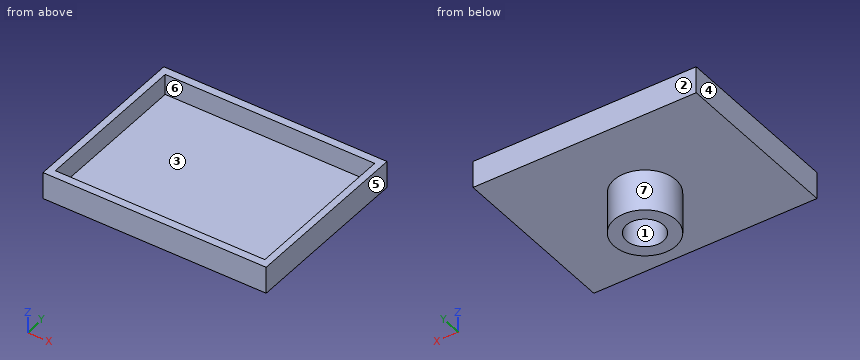
from build123d import *

# Parameters (mm, degrees)
ESQUISSE1_R             = 7.5
ESQUISSE1_R_2           = 4.5
BOSS_EXTRU_1_DEPTH      = 10
ESQUISSE2_W             = 54
ESQUISSE2_H             = 42
BOSS_EXTRU_2_DEPTH      = 6.5
ESQUISSE4_W             = 50.7
ESQUISSE4_H             = 38.2
ENL_V_MAT_EXTRU_2_DEPTH = 5


with BuildPart() as part:
    # Esquisse1 → Boss.-Extru.1 (new body)
    with BuildSketch(Plane.XY):
        Circle(ESQUISSE1_R)
        Circle(ESQUISSE1_R_2, mode=Mode.SUBTRACT)
    extrude(amount=BOSS_EXTRU_1_DEPTH)

    # Esquisse2 → Boss.-Extru.2 (add)
    with BuildSketch(Plane.XY.offset(10)):
        Rectangle(ESQUISSE2_W, ESQUISSE2_H)
    extrude(amount=BOSS_EXTRU_2_DEPTH)

    # Esquisse4 → Enlèv. mat.-Extru.2 (cut)
    with BuildSketch(Plane.XY.offset(16.5)):
        Rectangle(ESQUISSE4_W, ESQUISSE4_H)
    extrude(amount=-ENL_V_MAT_EXTRU_2_DEPTH, mode=Mode.SUBTRACT)


solid = part.part
Can you work these out from the model? Positions are in its coordinate system, mm. Face numbers are marked on the shaded views. A direction names the side the tool comes from. Round coordinates to 2 decimals unless told otherwise and drop trailing zeros. Order: outer loops, then holes, each group sorted by start corner. A loop starts at its lowest first (then second) coordinate and runs counter-clockwise, first axis right, second up. Notation, with made-up numbers: (-28.5, 23.5) -> (5.5, 23.5) arc R5 cw to (5.5, 30.5) -> close; hole circle Ø11 at (32, -31.75). An arc over 180 degrees is marked (long way). Write each question's results on one line, items separated by ' | '. Start each with the question number.
Item 1: If we section it at D-D, the plane y = -12.5: Write out the boundary of the cut face in (x, z), then the cut area to 3 significant figures.
Item 2: Which directions (+Z, -Z, +X, -X, +Y, -Y) give clear straight access to the entire face, cutting with the end or side of a thin tool? Please do the marked faces 5, 6 and 7.
Item 3: If we section it at A-A, the plane y = 0: Write out the boundary of the cut face in (x, z), then the cut area to 4 significant figures.
Item 4: Thinking about a two-plate mould opening in Y: for the marked faces 1, 2, 3 and 4, which applies, +Y half, -Y half, draft (parallel to the pull), parting line (faces both ways), or undercut?
Item 5: Please list where these lines run through material, in increasing order: L1, parallel to Y at x = 0, z = 8; L2, parallel to X at y = 8.5, z = 15.5; L3, parallel to Z at x = -12.5, y = -8.
Item 6: If we section it at B-B, the plane z = 13: Write out the boundary of the cut face in (x, y), then the cut area to 3 significant figures.
Item 7: Will these pins go through, and if not, where does the flat tip stop? pin 1 (1.5 mm diameter, centred on x = -20.5, y = -3.5, fed in from +Z); pin 2 (4 mm diameter, centred on x = 13.5, y = -13, fed in from -Z).
Item 8: If we section it at C-C, the plane x = 21: Write out the boundary of the cut face in (y, z).
Results:
1) outline: (-27, 10) -> (27, 10) -> (27, 16.5) -> (25.35, 16.5) -> (25.35, 11.5) -> (-25.35, 11.5) -> (-25.35, 16.5) -> (-27, 16.5) -> close | area: 97.5 mm2
2) face 5: +Z, -Z, +X, +Y, -Y | face 6: +Z | face 7: -Z
3) outline: (-27, 10) -> (-7.5, 10) -> (-7.5, 0) -> (-4.5, 0) -> (-4.5, 10) -> (4.5, 10) -> (4.5, 0) -> (7.5, 0) -> (7.5, 10) -> (27, 10) -> (27, 16.5) -> (25.35, 16.5) -> (25.35, 11.5) -> (-25.35, 11.5) -> (-25.35, 16.5) -> (-27, 16.5) -> close | area: 157.5 mm2
4) face 1: undercut | face 2: +Y half | face 3: undercut | face 4: draft
5) L1: y = -7.5 to -4.5, 4.5 to 7.5 | L2: x = -27 to -25.35, 25.35 to 27 | L3: z = 10 to 11.5
6) outline: (-27, -21) -> (27, -21) -> (27, 21) -> (-27, 21) -> close; hole (-25.35, -19.1) -> (25.35, -19.1) -> (25.35, 19.1) -> (-25.35, 19.1) -> close | area: 331 mm2
7) pin 1: stops at z = 11.5 | pin 2: stops at z = 10
8) outline: (-21, 10) -> (21, 10) -> (21, 16.5) -> (19.1, 16.5) -> (19.1, 11.5) -> (-19.1, 11.5) -> (-19.1, 16.5) -> (-21, 16.5) -> close
